Work out the finished part from the listing and answer in its coordinate system (mm). Give positions to 0.01 mm unless a question says otherwise; leave off trailing zeros. Order: outer loops, then holes, each group sorted by start corner. A loop starts at its lowest first (then second) coordinate and runs counter-clockwise, first axis right, second up. Notation, with made-up numbers: (62, 74) - (106, 74) arc R17 ccw to (106, 97) - close; hole circle Ø7 at (-28, 52). An arc over 180 degrees is marked (long way). Write each question's results on one line, items separated by ' | '.
Autodesk Inventor part; units mm, degrees
ref_plane "YZ Plane" through (0, 0, 0) normal (1, 0, 0) x (0, 1, 0)
ref_plane "XZ Plane" through (0, 0, 0) normal (0, 1, 0) x (-1, 0, 0)
ref_plane "XY Plane" through (0, 0, 0) normal (0, 0, 1) x (1, 0, 0)
sketch "Sketch1" plane through (0, 0, 0) normal (0, 0, 1) x (1, 0, 0)
  line L0 (0, 0) -> (0, 101.6)
  line L1 (0, 101.6) -> (101.6, 101.6)
  line L2 (101.6, 101.6) -> (101.6, 0)
  line L3 (101.6, 0) -> (0, 0)
  circle A0 centre (12.7, 92.4868) radius 1.5875
  circle A1 centre (12.7, 73.555) radius 1.5875
  circle A2 centre (12.7, 57.3937) radius 1.5875
  circle A3 centre (12.7, 43.772) radius 1.5875
  circle A4 centre (12.7, 31.3047) radius 1.5875
  circle A5 centre (12.7, 18.1448) radius 1.5875
  circle A6 centre (12.7, 5.9084) radius 1.5875
  circle A7 centre (88.9, 92.4868) radius 1.5875
  circle A8 centre (88.9, 73.555) radius 1.5875
  circle A9 centre (88.9, 57.3937) radius 1.5875
  circle A10 centre (88.9, 39.5628) radius 1.5875
  circle A11 centre (88.9, 31.3047) radius 1.5875
  circle A12 centre (88.9, 18.1448) radius 1.5875
  circle A13 centre (88.9, 5.9084) radius 1.5875
  circle A14 centre (50.8, 81.1516) radius 3.175
  circle A15 centre (30.9641, 70.6359) radius 3.175
  circle A16 centre (30.985, 30.985) radius 3.175
  circle A17 centre (50.8, 14.339) radius 3.175
  circle A18 centre (70.615, 30.985) radius 3.175
  circle A19 centre (68.3905, 68.3905) radius 3.175
  line L4 (0, 101.6) -> (101.6, 0) construction
  line L5 (0, 0) -> (101.6, 101.6) construction
  line L6 (0, 50.8) -> (101.6, 50.8) construction
  line L7 (50.8, 50.8) -> (50.8, 101.6) construction
  line L8 (50.8, 50.8) -> (50.8, 0) construction
  dimension "d0" = 101.6
  dimension "d1" = 101.6
  dimension "d2" = 3.175
  dimension "d3" = 3.175
  dimension "d4" = 3.175
  dimension "d5" = 3.175
  dimension "d6" = 3.175
  dimension "d7" = 3.175
  dimension "d8" = 3.175
  dimension "d9" = 12.7
  dimension "d10" = 12.7
  dimension "d11" = 12.7
  dimension "d12" = 12.7
  dimension "d13" = 12.7
  dimension "d14" = 12.7
  dimension "d15" = 12.7
  dimension "d18" = 3.175
  dimension "d19" = 3.175
  dimension "d20" = 3.175
  dimension "d21" = 3.175
  dimension "d22" = 3.175
  dimension "d23" = 3.175
  dimension "d24" = 3.175
  dimension "d25" = 12.7
  dimension "d26" = 12.7
  dimension "d27" = 12.7
  dimension "d28" = 12.7
  dimension "d29" = 12.7
  dimension "d30" = 12.7
  dimension "d31" = 12.7
  dimension "d58" = 6.35
  dimension "d59" = 6.35
  dimension "d60" = 6.35
  dimension "d61" = 6.35
  dimension "d62" = 6.35
  dimension "d63" = 6.35
extrude "Extrusion1" add sketch "Sketch1" against normal blind 25.4 contours L0 L1 L2 L3 | A7 | A8 | A9 | A10 | A11 | A12 | A13 | A14 | A15 | A16 | A17 | A18 | A19
extrude "Extrusion2" cut sketch "Sketch1" against normal blind 25.4 contours A7
extrude "Extrusion3" cut sketch "Sketch1" against normal blind 25.4 contours A8
extrude "Extrusion4" cut sketch "Sketch1" against normal blind 25.4 contours A9
extrude "Extrusion5" cut sketch "Sketch1" against normal blind 25.4 contours A10
extrude "Extrusion6" cut sketch "Sketch1" against normal blind 25.4 contours A11
extrude "Extrusion7" cut sketch "Sketch1" against normal blind 25.4 contours A12
extrude "Extrusion8" cut sketch "Sketch1" against normal blind 25.4 contours A13
extrude "Extrusion9" cut sketch "Sketch1" against normal blind 25.4 contours A15
extrude "Extrusion10" cut sketch "Sketch1" against normal blind 25.4 contours A16
extrude "Extrusion11" cut sketch "Sketch1" against normal blind 25.4 contours A14
extrude "Extrusion12" cut sketch "Sketch1" against normal blind 25.4 contours A19
extrude "Extrusion13" cut sketch "Sketch1" against normal blind 25.4 contours A18
extrude "Extrusion14" cut sketch "Sketch1" against normal blind 25.4 contours A17
properties part number "PopQuiz"
1. A cutting plane is placed at A-A, the plane x = 88.9. State how many separate pieces and enclosed holes the cut face has, then the cut area to 3 significant figures.
Answer list:
separate pieces: 8 | enclosed holes: 0 | area: 2,020 mm^2
2. Determine the mould class of faces 1 (the face through (32.692, 33.662, -12.522)), 2 (the face through (0, 50, -13)), 3 (the face through (71.42, 69.34, -12.52)), 4 (the face through (50, 52, -25.4)) for opening direction X: +X half, -X half, draft (parallel to the pull), parting line (faces both ways), or undercut.
Answer list:
face 1: undercut | face 2: -X half | face 3: undercut | face 4: draft
3. Given P1, Ø4, axis at x = 51.5, y = 85, coming from the +Z side, flat-ended and moving along its own axis, determine where the tip first touches the part or whether it passes through.
Answer list:
P1: z = 0
4. Straight lines are drawn through the part: line 1 (X direction, y = 18, z = -15.25); line 2 (X direction, y = 5.5, z = -14.5); line 3 (X direction, y = 79.5, z = -5.5). For each, find the intervals that lie inside material, in ascending order. Write a range as [from, to].
Answer list:
line 1: [0, 11.12], [14.28, 87.32], [90.48, 101.6] | line 2: [0, 11.17], [14.23, 87.37], [90.43, 101.6] | line 3: [0, 48.09], [53.51, 101.6]
5. A cutting plane is placed at B-B, the plane x = 50.8. Write down the section's boundary in (y, z), then the cut area to 3 significant figures.
Answer list:
outline: (0, -25.4) - (11.16, -25.4) - (11.16, 0) - (0, 0) - close; (17.51, -25.4) - (77.98, -25.4) - (77.98, 0) - (17.51, 0) - close; (84.33, -25.4) - (101.6, -25.4) - (101.6, 0) - (84.33, 0) - close | area: 2,260 mm^2
